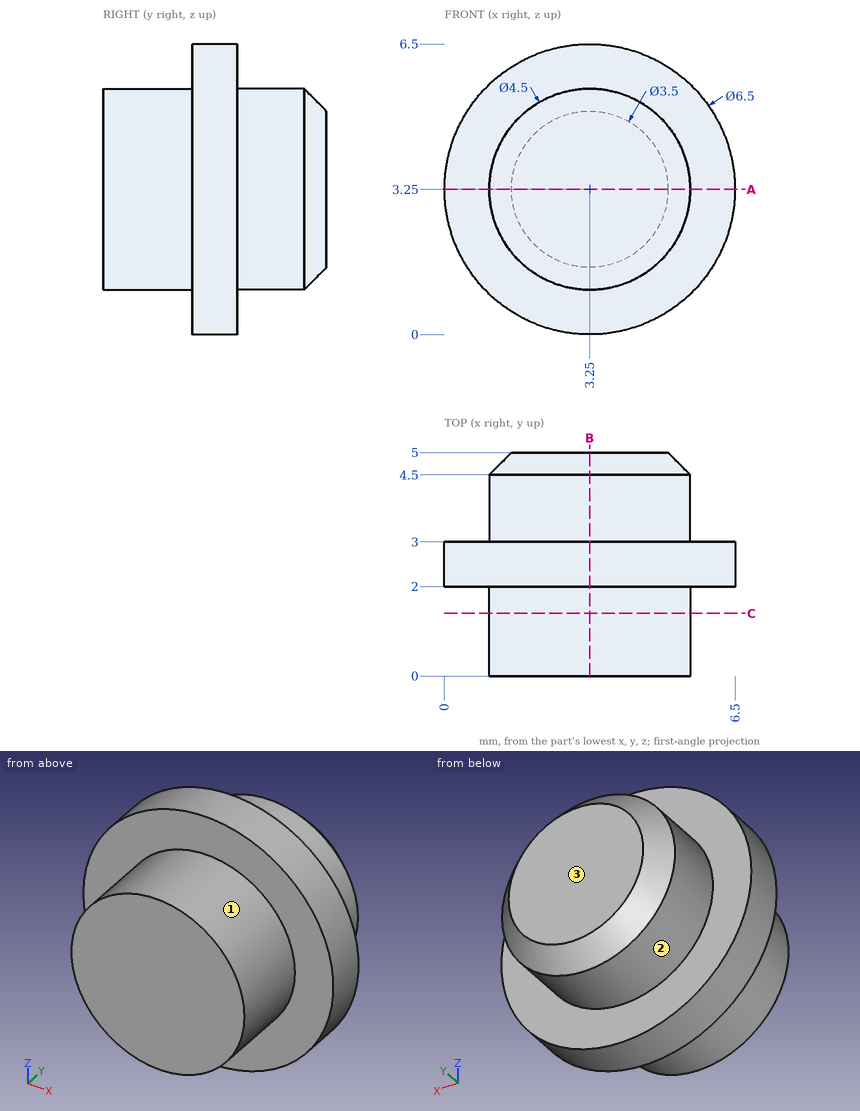
Here's the drawing with two shaded views (mm, measured from the low corner). I have some questions. A direction names the side the tool comes from. Coordinates: 2 decimals unless noted, no trailing zeros. Loops run counter-clockwise (first coordinate to the right, second up) from the corner with the lowest first, then second, coordinate; pieces in that order, holes last. Notation, with made-up numbers: (34, 34) -> (92, 34) arc R14 ccw to (92, 38) -> close; hole circle Ø2 at (84.5, -8.75). An arc over 180 degrees is marked (long way). Answer in a Markdown table with one row per item.
(1) Imagine slicing it at C-C (y = 1.4). List the corners of the cut face in (x, z) for me.
Results found:
| item | result |
|---|---|
| outline | circle Ø4.5 at (3.25, 3.25) |
(2) Imagine slicing it at A-A (z = 3.25). List the corners of the cut face in (x, y) for me, plus the area to 4 significant figures.
Results found:
| item | result |
|---|---|
| outline | (0, 2) -> (1, 2) -> (1, 0) -> (5.5, 0) -> (5.5, 2) -> (6.5, 2) -> (6.5, 3) -> (5.5, 3) -> (5.5, 4.5) -> (5, 5) -> (1.5, 5) -> (1, 4.5) -> (1, 3) -> (0, 3) -> close |
| area | 24.25 mm^2 |
(3) If I drill on probe 1 along Y at (x, z) = (5, 1.25); probe 2 along Z at (x, y) = (5.75, 2.4); probe 3 along Z at (x, y) = (3, 1.7), over which ranges is the centre line in solid material (lowest first)?
Results found:
| item | result |
|---|---|
| probe 1 | y = 2 to 3 |
| probe 2 | z = 1.17 to 5.33 |
| probe 3 | z = 1.01 to 5.49 |
(4) Imagine slicing it at B-B (x = 3.25). List the corners of the cut face in (y, z) for me.
Results found:
| item | result |
|---|---|
| outline | (0, 1) -> (2, 1) -> (2, 0) -> (3, 0) -> (3, 1) -> (4.5, 1) -> (5, 1.5) -> (5, 5) -> (4.5, 5.5) -> (3, 5.5) -> (3, 6.5) -> (2, 6.5) -> (2, 5.5) -> (0, 5.5) -> close |
(5) For the marked faces 1, 2 and 3, which set-ups out of +Z, -Z, +X, -X, +Y, -Y let a thin tool reach every point of the face, with its end or its side?
Results found:
| item | result |
|---|---|
| face 1 | -Y |
| face 2 | +Y |
| face 3 | +Z, -Z, +X, -X, +Y |
